from build123d import *

# Parameters (mm, degrees)
SKETCH2_R           = 7.9
BOSS_EXTRUDE1_DEPTH = 5
SKETCH3_R           = 10
BOSS_EXTRUDE2_DEPTH = 100
SKETCH4_R           = 6
CUT_EXTRUDE2_DEPTH  = 200
SKETCH5_R           = 8
BOSS_EXTRUDE3_DEPTH = 5
CUT_EXTRUDE3_START  = -5
SKETCH6_R           = 6
CUT_EXTRUDE3_DEPTH  = 5
BOSS_EXTRUDE5_START = 5
SKETCH10_R          = 8
BOSS_EXTRUDE5_DEPTH = 5
CUT_EXTRUDE5_START  = -10
SKETCH11_R          = 6
CUT_EXTRUDE5_DEPTH  = 10
SKETCH12_R          = 2
CUT_EXTRUDE6_DEPTH  = 20
SKETCH13_R          = 2
CUT_EXTRUDE7_DEPTH  = 20
CUT_EXTRUDE9_START  = -10
SKETCH15_R          = 8
CUT_EXTRUDE9_DEPTH  = 10


with BuildPart() as part:
    # Sketch2 → Boss-Extrude1 (new body)
    with BuildSketch(Plane(origin=(0, 0, 0), x_dir=(1, 0, 0), z_dir=(0, 1, 0))):
        with Locations(Location((0, 0, 0), (0, 0, 270))):
            Circle(SKETCH2_R)
    extrude(amount=BOSS_EXTRUDE1_DEPTH)

    # Sketch3 → Boss-Extrude2 (add)
    with BuildSketch(Plane(origin=(0, 5, 0), x_dir=(1, 0, 0), z_dir=(0, 1, 0))):
        with Locations(Location((0, 0, 0), (0, 0, 270))):
            Circle(SKETCH3_R)
    extrude(amount=BOSS_EXTRUDE2_DEPTH)

    # Sketch4 → Cut-Extrude2 (cut)
    with BuildSketch(Plane(origin=(0, 105, 0), x_dir=(1, 0, 0), z_dir=(0, 1, 0))):
        with Locations(Location((0, 0, 0), (0, 0, 270))):
            Circle(SKETCH4_R)
    extrude(amount=-CUT_EXTRUDE2_DEPTH, mode=Mode.SUBTRACT)

    # Sketch5 → Boss-Extrude3 (add)
    with BuildSketch(Plane(origin=(0, 0, 0), x_dir=(-1, 0, 0), z_dir=(0, -1, 0))):
        with Locations(Location((0, 0, 0), (0, 0, 90))):
            Circle(SKETCH5_R)
    extrude(amount=-BOSS_EXTRUDE3_DEPTH)

    # Sketch6 → Cut-Extrude3 (cut)
    with BuildSketch(Plane(origin=(0, 0, 0), x_dir=(-1, 0, 0), z_dir=(0, -1, 0)).offset(CUT_EXTRUDE3_START)):
        with Locations(Location((0, 0, 0), (0, 0, 270))):
            Circle(SKETCH6_R)
    extrude(amount=CUT_EXTRUDE3_DEPTH, mode=Mode.SUBTRACT)

    # Sketch10 → Boss-Extrude5 (add)
    with BuildSketch(Plane(origin=(0, 0, 0), x_dir=(-1, 0, 0), z_dir=(0, -1, 0)).offset(BOSS_EXTRUDE5_START)):
        with Locations(Location((0, 0, 0), (0, 0, 90))):
            Circle(SKETCH10_R)
    extrude(amount=-BOSS_EXTRUDE5_DEPTH)

    # Sketch11 → Cut-Extrude5 (cut)
    with BuildSketch(Plane(origin=(0, -5, 0), x_dir=(-1, 0, 0), z_dir=(0, -1, 0)).offset(CUT_EXTRUDE5_START)):
        with Locations(Location((0, 0, 0), (0, 0, 270))):
            Circle(SKETCH11_R)
    extrude(amount=CUT_EXTRUDE5_DEPTH, mode=Mode.SUBTRACT)

    # Sketch12 → Cut-Extrude6 (cut)
    with BuildSketch(Plane.XY.offset(10)):
        Circle(SKETCH12_R)
    extrude(amount=-CUT_EXTRUDE6_DEPTH, mode=Mode.SUBTRACT)

    # Sketch13 → Cut-Extrude7 (cut)
    with BuildSketch(Plane.XY.offset(10)):
        with Locations(Location((0, 100, 0), (0, 0, 270.000000021))):
            Circle(SKETCH13_R)
    extrude(amount=-CUT_EXTRUDE7_DEPTH, mode=Mode.SUBTRACT)

    # Sketch15 → Cut-Extrude9 (cut)
    with BuildSketch(Plane(origin=(0, 105, 0), x_dir=(1, 0, 0), z_dir=(0, 1, 0)).offset(CUT_EXTRUDE9_START)):
        with Locations(Location((0, 0, 0), (0, 0, 90))):
            Circle(SKETCH15_R)
    extrude(amount=CUT_EXTRUDE9_DEPTH, mode=Mode.SUBTRACT)


solid = part.part
Part model, mm, in its own coordinate system. A direction names the side the tool comes from. Give positions to 0.01 mm unless a question says otherwise; leave off trailing zeros. Write each loop counter-clockwise with the first axis right and the second up, starting at its lowest first coordinate (ties: lowest second). Pieces come first, ordered by that corner, then holes.
1) Which spindle directions (+Z, -Z, +X, -X, +Y, -Y) get a long thin tool onto all of the face, cutting with end or side? Do faces 4 (the face through (3.06, 99.93, -7.39)), 5 (the face through (-3.06, -0.07, -7.39)), 6 (the face through (1.908, 0.601, -6.812)). Say none if no direction does.
Resolved:
face 4: +Y
face 5: -Y
face 6: +Z, -Z
2) Two-plate mould, pull along Y, no slides. Class faces 1 (the face through (-6, 95, 2)), 2 (the face through (8.2, 5, 0)), 3 (the face through (1.352, 101.474, 8.889)): released by +Y, released by -Y, zero draft, split by the parting line, or undercut.
Resolved:
face 1: released by +Y
face 2: released by -Y
face 3: undercut
3) Cut at A-A on x = 0. State how many separate pieces and enclosed holes the cut face has, then the cut area to 3 significant figures.
Resolved:
separate pieces: 6
enclosed holes: 0
area: 768 mm2
4) Pin check, flat tips, straight feed: pin 1 (4.5 mm diameter, centred on x = 0, y = 100, fed in from -Z); pin 2 (6.5 mm diameter, centred on x = 0, y = 0, fed in from -Z); pin 3 (10 mm diameter, centred on x = 7, y = 41.5, fed in from +Z); pin 4 (1.5 mm diameter, centred on y = 11.5, z = -4, fed in from -X). Stop position of each tip, or through.
Resolved:
pin 1: stops at z = -10
pin 2: stops at z = -8
pin 3: stops at z = 9.8
pin 4: stops at x = -9.46
5) Cut at C-C on z = -1.5. Write the cut outline in (x, y), then the cut area to 3 significant figures.
Resolved:
outline: (-9.89, 5) - (-7.86, 5) - (-7.86, -5) - (-5.81, -5) - (-5.81, 95) - (-7.86, 95) - (-7.86, 105) - (-9.89, 105) - close; (5.81, -5) - (7.86, -5) - (7.86, 5) - (9.89, 5) - (9.89, 105) - (7.86, 105) - (7.86, 95) - (5.81, 95) - close
area: 815 mm2
6) Probe L1, parallel to X at y = 30, z = 0.25; L2, parallel to Z at x = -3.75, y = 53; L3, parallel to Z at x = 2.25, y = 99. List the from-to ranges inside material, lowest first.
Resolved:
L1: x = -10 to -5.99, 5.99 to 10
L2: z = -9.27 to -4.68, 4.68 to 9.27
L3: z = -9.74 to -7.68, 7.68 to 9.74
7) Cut at D-D on x = -4.25. Write the cut outline in (y, z), then the cut area to 3 significant figures.
Resolved:
outline: (-5, -6.78) - (5, -6.78) - (5, -9.05) - (105, -9.05) - (105, -6.78) - (95, -6.78) - (95, -4.24) - (-5, -4.24) - close; (-5, 4.24) - (95, 4.24) - (95, 6.78) - (105, 6.78) - (105, 9.05) - (5, 9.05) - (5, 6.78) - (-5, 6.78) - close
area: 963 mm2
8) Cut at B-B on y = 0. Write the cut outline in (x, z), then the cut area to 3 significant figures.
Resolved:
outline: (-2, -7.75) - (-2, -5.66) arc R6 cw to (-2, 5.66) - (-2, 7.75) arc R8 ccw to start; (2, -7.75) arc R8 ccw to (2, 7.75) - (2, 5.66) arc R6 cw to (2, -5.66) - close
area: 71.7 mm2
